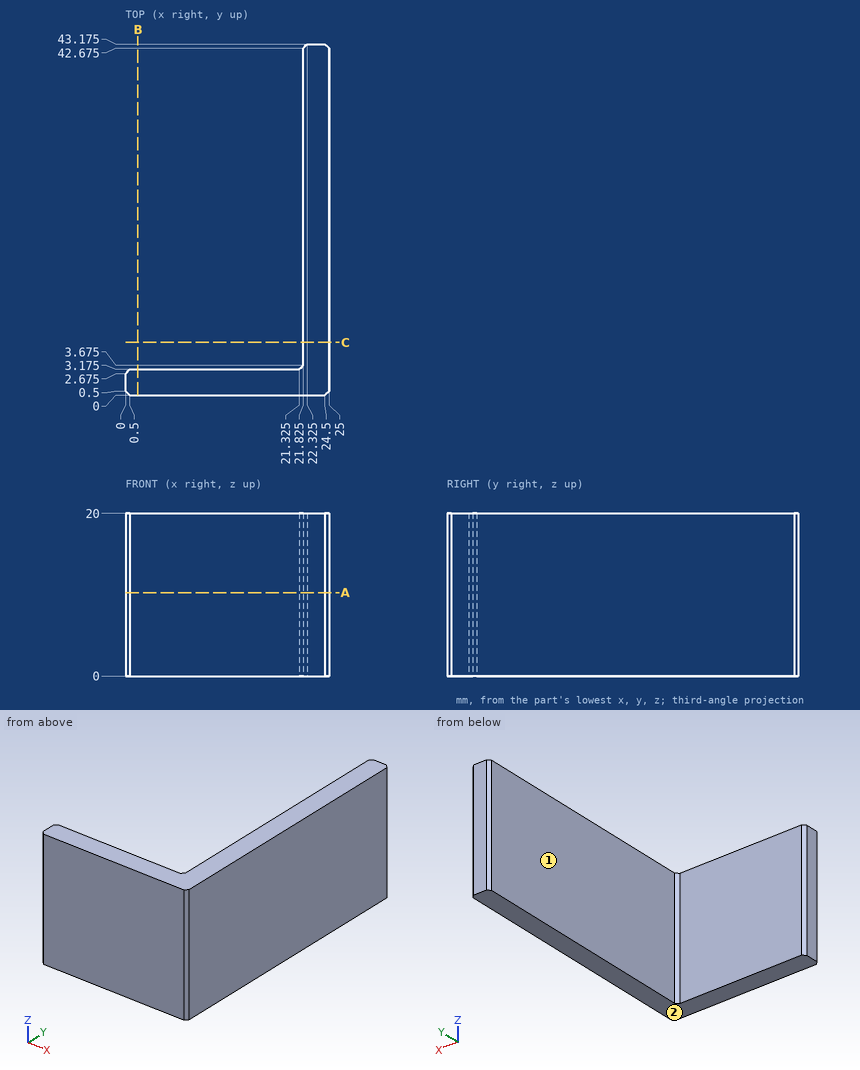
Could you check a few things on this drawing? It's one solid part, dimensions in mm from its lowest x, y, z. A direction names the side the tool comes from. Give positions to 0.01 mm unless a question says otherwise; leave off trailing zeros. Order: outer loops, then holes, each group sorted by start corner. A loop starts at its lowest first (then second) coordinate and runs counter-clockwise, first axis right, second up. Notation, with made-up numbers: (40.5, 49.25) - (81.5, 49.25) arc R20 ccw to (81.5, 64.25) - close; hole circle Ø5 at (82, 74). An arc over 180 degrees is marked (long way). Return JSON: item names as keys, results as strings. Group by question number.
Q1. Suppose I cut it at C-C, the plane y = 6.5. Please give me the cut outline in (x, z) (3 decimals).
Q2. Please list where these lines run through material, in increasing order: line 1 along X through (y, z) = (5, 11.75) (3 decimals); line 2 along Y through (x, z) = (20.5, 4.25) (3 decimals). Write a range as [from, to].
Q3. Which directions (+Z, -Z, +X, -X, +Y, -Y) give clear straight access to the entire face, cutting with the end or side of a thin tool? Please do the marked faces 1 and 2.
Q4. Will these pins go through, and if not, where does the flat tip stop? pin 1 Ø4 at (y, z) = (7, 9.5) entering from -X (3 decimals); pin 2 Ø8 at (x, z) = (20, 9.5) entering from +Y (3 decimals); pin 3 Ø1.5 at (x, z) = (20.5, 15) entering from +Y (3 decimals).
Q5. Suppose I cut it at B-B, the plane x = 1.5. Please give me the cut outline in (y, z) (3 decimals), and give its area (3 significant figures).
Q6. Suppose I cut it at A-A, the plane z = 10.25. Please give me the cut outline in (x, y) (3 decimals), and give its area (3 significant figures).
Resolved:
{
 "1": {"outline": "(21.825, 0) - (25, 0) - (25, 20) - (21.825, 20) - close"},
 "2": {"line 1": "x = [21.825, 25]", "line 2": "y = [0, 3.175]"},
 "3": {"face 1": "+Z, -Z, -X, +Y", "face 2": "-Z, +X, -X, +Y, -Y"},
 "4": {"pin 1": "stops at x = 21.825", "pin 2": "stops at y = 43.175", "pin 3": "stops at y = 3.175"},
 "5": {"outline": "(0, 0) - (3.175, 0) - (3.175, 20) - (0, 20) - close", "area": "63.5 mm2"},
 "6": {"outline": "(0, 0.5) - (0.5, 0) - (24.5, 0) - (25, 0.5) - (25, 42.675) - (24.5, 43.175) - (22.325, 43.175) - (21.825, 42.675) - (21.825, 3.675) - (21.325, 3.175) - (0.5, 3.175) - (0, 2.675) - close", "area": "206 mm2"}
}
